```python
from build123d import *

# Parameters (mm, degrees)
SKETCH1_W                                      = 158.75
SKETCH1_H                                      = 50.8
BOSS_EXTRUDE1_DEPTH                            = 1.5875
CSK_FOR_M4_FLAT_HEAD_MACHINE_SCREW1_AT_2_COUNT = 2
CSK_FOR_M4_FLAT_HEAD_MACHINE_SCREW1_AT_2_PITCH = 25.4
CSK_FOR_M4_FLAT_HEAD_MACHINE_SCREW1_AT_3_COUNT = 2
CSK_FOR_M4_FLAT_HEAD_MACHINE_SCREW1_AT_3_PITCH = 98.578509321
CSK_FOR_M4_FLAT_HEAD_MACHINE_SCREW1_AT_4_COUNT = 2
CSK_FOR_M4_FLAT_HEAD_MACHINE_SCREW1_AT_4_PITCH = 95.25


with BuildPart() as part:
    # Sketch1 → Boss-Extrude1 (new body)
    with BuildSketch(Plane.XY):
        with Locations((-79.375, 25.4)):
            Rectangle(SKETCH1_W, SKETCH1_H)
    extrude(amount=BOSS_EXTRUDE1_DEPTH)

    # Sketch2 → CSK for M4 Flat Head Machine Screw1 (revolve, cut)
    with BuildSketch(Plane(origin=(-127, 37.973, 1.5875), x_dir=(0, -1, 0), z_dir=(1, 0, 0))):
        Polygon((0, 0), (0, 1.5875), (2.25, 1.5875), (2.25, 2.45), (4.7, 0), align=None)
    csk_for_m4_flat_head_machine_screw1 = revolve(axis=Axis((-127, 37.973, 7.9375), (0, 0, -1)), mode=Mode.SUBTRACT)

    # CSK for M4 Flat Head Machine Screw1 at 2: CSK for M4 Flat Head Machine Screw1 ×2
    with Locations(*[(0, -i * CSK_FOR_M4_FLAT_HEAD_MACHINE_SCREW1_AT_2_PITCH, 0) for i in range(1, CSK_FOR_M4_FLAT_HEAD_MACHINE_SCREW1_AT_2_COUNT)]):
        add(csk_for_m4_flat_head_machine_screw1, mode=Mode.SUBTRACT)

    # CSK for M4 Flat Head Machine Screw1 at 3: CSK for M4 Flat Head Machine Screw1 ×2
    with Locations(*[Vector(0.9662349396012463, -0.25766265056033233, 0) * (i * CSK_FOR_M4_FLAT_HEAD_MACHINE_SCREW1_AT_3_PITCH) for i in range(1, CSK_FOR_M4_FLAT_HEAD_MACHINE_SCREW1_AT_3_COUNT)]):
        add(csk_for_m4_flat_head_machine_screw1, mode=Mode.SUBTRACT)

    # CSK for M4 Flat Head Machine Screw1 at 4: CSK for M4 Flat Head Machine Screw1 ×2
    with Locations(*[(i * CSK_FOR_M4_FLAT_HEAD_MACHINE_SCREW1_AT_4_PITCH, 0, 0) for i in range(1, CSK_FOR_M4_FLAT_HEAD_MACHINE_SCREW1_AT_4_COUNT)]):
        add(csk_for_m4_flat_head_machine_screw1, mode=Mode.SUBTRACT)


solid = part.part
```
Could you check a few things on this model? Use its own coordinates, in mm. Round coordinates to 2 decimals unless told otherwise and drop trailing zeros. Write each loop counter-clockwise with the first axis right and the second up, starting at its lowest first coordinate (ties: lowest second). Pieces come first, ordered by that corner, then holes. Notation, with made-up numbers: M 85,-36.5 L 129,-36.5 A8 ccw 129,-31.5 Z; hole C 24.5,-30.5 d3. An arc over 180 degrees is marked long. Answer in a Markdown table with one row per item. Add a question column.
Q1. Imagine slicing it at A-A (z = 0.75). Give the number of separate pieces and of enclosed holes in the cut face, then the cut area to 3 significant figures.
Q2. Imagine slicing it at B-B (x = -127). Please give me the cut outline in (y, z), then the cut area to 3 significant figures.
Q3. Will this pin go through, and if not, where does the flat tip stop? pin 1 Ø12 at (x, y) = (-51.5, 10.5) entering from -Z.
Q4. If I drill on line 1 (X direction, y = 41, z = 0.95); line 2 (Y direction, x = -34.5, z = 0.35); line 3 (X direction, y = 10, z = 0.9), over which ranges is the centre line in solid material (lowest first)? Write a range as from..to.
Values:
| question | item | result |
|---|---|---|
| 1 | separate pieces | 1 |
| 1 | enclosed holes | 4 |
| 1 | area | 7,880 mm^2 |
| 2 | outline | M 0,0 L 9.46,0 L 7.87,1.59 L 0,1.59 Z; M 15.69,0 L 34.86,0 L 33.27,1.59 L 17.27,1.59 Z; M 41.09,0 L 50.8,0 L 50.8,1.59 L 42.67,1.59 Z |
| 2 | area | 55.8 mm^2 |
| 3 | pin 1 | z = 0 |
| 4 | line 1 | -158.75..-129.71, -124.29..-34.46, -29.04..0 |
| 4 | line 2 | 0..10.47, 14.68..35.87, 40.08..50.8 |
| 4 | line 3 | -158.75..-130.08, -123.92..-34.83, -28.67..0 |
